Source: CAD feature listing. Evaluate the final solid. Frame: model axes, mm. A direction names the side the tool comes from. Round coordinates to 2 decimals unless told otherwise and drop trailing zeros. Loops run counter-clockwise (first coordinate to the right, second up) from the corner with the lowest first, then second, coordinate; pieces in that order, holes last. Notation, with made-up numbers: M -17.5,-14.75 L 40.5,-14.75 A20 ccw 40.5,17.25 Z; hole C 22,-22.75 d8. An arc over 180 degrees is marked long. Write each question's results on one line, items separated by ' | '. Start each with the question number.
1. Set-up query: faces 1 (the flat face through (6, -61.413, -4)), 2 (the flat face through (12, 36.087, -1)), 3 (the flat face through (-9.516, -25, 4)). Return all of +Z, -Z, +X, -X, +Y, -Y with unobstructed straight access to the full face (end or side cutting, diameter ignored); none if empty.
2. Draft query along Z for faces 4 (the flat face through (5.106, -63.857, 4.056)), 5 (the flat face through (20.484, -55, 7)), 6 (the flat face through (5.694, -19.969, 3.944)). Return one class per face: released by +Z, released by -Z, zero draft, split by the parting line, or undercut.
3. Ray query, line 1 (Y direction, x = -7, z = -0.25); line 2 (Y direction, x = 11.5, z = -1.5); line 3 (X direction, y = -0.5, z = -0.5). Return the intervals inside material, ascending.
4. Section C-C on y = 10.5. Output: boundary loops of the cut face in (x, z), and give its area (3 significant figures).
5. Section D-D on x = -4. Give the number of separate pieces and of enclosed holes in the cut face, and give its area (3 significant figures).
6. Section B-B on x = -10.5. Output: boundary loops of the cut face in (y, z), and give its area (3 significant figures).
7. Contact query for flat-ended pins moving along their axis: pin 1 Ø6.5 at (y, z) = (7.5, 4) entering from -X; pin 2 Ø12.5 at (x, y) = (12.5, -22) entering from -Z; pin 3 Ø6.5 at (y, z) = (-25.5, 5.5) entering from +X. Output: stop coordinate, or through.
8. Section A-A on z = -3.25. Output: boundary loops of the cut face in (x, y).
from build123d import *

# Parameters (mm, degrees)
SKETCH1_W               = 54
SKETCH1_H               = 104
SKETCH1_W_2             = 30
SKETCH1_H_2             = 80
BOSS_EXTRUDE1_DEPTH     = 8
CHAMFER1_SIZE           = 8
SKETCH2_W               = 54
SKETCH2_H               = 104
SKETCH2_W_2             = 50
SKETCH2_H_2             = 100
BOSS_EXTRUDE2_DEPTH     = 2
SKETCH3_W               = 44
SKETCH3_H               = 94
SKETCH3_W_2             = 41
SKETCH3_H_2             = 91
BOSS_EXTRUDE3_DEPTH     = 9
CUT_EXTRUDE1_REACH      = 106.581
SKETCH4_W               = 17
SKETCH4_H               = 1
CUT_EXTRUDE2_DEPTH      = 110.326033519
CUT_EXTRUDE2_DEPTH_BACK = 2
BOSS_EXTRUDE4_REACH     = 82.357


with BuildPart() as part:
    # Sketch1 → Boss-Extrude1 (new body)
    with BuildSketch(Plane.XY):
        with Locations((5.483558994, -15.912959381)):
            Rectangle(SKETCH1_W, SKETCH1_H)
        with Locations((5.483558994, -15.912959381)):
            Rectangle(SKETCH1_W_2, SKETCH1_H_2, mode=Mode.SUBTRACT)
    extrude(amount=BOSS_EXTRUDE1_DEPTH)

    # Chamfer1
    chamfer1_edges = [part.edges().sort_by_distance(p)[0] for p in [
        (-21.516441006, -15.912959381, 8),
        (5.483558994, 36.087040619, 8),
        (32.483558994, -15.912959381, 8),
        (5.483558994, -67.912959381, 8),
    ]]
    chamfer(chamfer1_edges, length=CHAMFER1_SIZE - 0.0001)  # a hair under: the kernel refuses the full size

    # Sketch2 → Boss-Extrude2 (add)
    with BuildSketch(Plane(origin=(0, 0, 0), x_dir=(-1, 0, 0), z_dir=(0, 0, -1))):
        with Locations((-5.483558994, -15.912959381)):
            Rectangle(SKETCH2_W, SKETCH2_H)
        with Locations((-5.483558994, -15.912959381)):
            Rectangle(SKETCH2_W_2, SKETCH2_H_2, mode=Mode.SUBTRACT)
    extrude(amount=BOSS_EXTRUDE2_DEPTH)

    # Sketch3 → Boss-Extrude3 (add)
    with BuildSketch(Plane(origin=(0, 0, 0), x_dir=(-1, 0, 0), z_dir=(0, 0, -1))):
        with Locations((-5.483558994, -15.912959381)):
            Rectangle(SKETCH3_W, SKETCH3_H)
        with Locations((-5.483558994, -15.912959381)):
            Rectangle(SKETCH3_W_2, SKETCH3_H_2, mode=Mode.SUBTRACT)
    extrude(amount=BOSS_EXTRUDE3_DEPTH)

    # Sketch4 → Cut-Extrude1 (cut, up to next)
    with BuildSketch(Plane(origin=(0, 31.087040619, 0), x_dir=(1, 0, 0), z_dir=(0, 1, 0)), mode=Mode.PRIVATE) as cut_extrude1_sk1:
        with Locations((5.483558994, 8.5)):
            Rectangle(SKETCH4_W, SKETCH4_H)
    cut_extrude1_tool1 = extrude(cut_extrude1_sk1.sketch, amount=-CUT_EXTRUDE1_REACH, mode=Mode.PRIVATE) & part.part
    add(cut_extrude1_tool1.solids().sort_by_distance((5.483559, 31.087041, -8.5))[0], mode=Mode.SUBTRACT)

    # Sketch5 → Cut-Extrude2 (cut, two sides: drawn at the far end of the back side and taken through both)
    with BuildSketch(Plane(origin=(0, 36.087040619, 0), x_dir=(1, 0, 0), z_dir=(0, 1, 0)).offset(-CUT_EXTRUDE2_DEPTH_BACK)):
        with BuildLine():
            Line((-76.690196685, 38.800488397), (-2.516441006, 2))
            ThreePointArc((-2.516441006, 2), (5.483558994, 0.124515497), (13.483558994, 2))
            Line((13.483558994, 2), (87.657314674, 38.800488397))
            Line((87.657314674, 38.800488397), (87.657314674, 204.402686182))
            Line((87.657314674, 204.402686182), (-76.690196685, 204.402686182))
            Line((-76.690196685, 204.402686182), (-76.690196685, 38.800488397))
        make_face()
    extrude(amount=CUT_EXTRUDE2_DEPTH + CUT_EXTRUDE2_DEPTH_BACK, mode=Mode.SUBTRACT)

    # Sketch6 → Boss-Extrude4 (add, up to next)
    with BuildSketch(Plane.ZY.offset(-20.483558994), mode=Mode.PRIVATE) as boss_extrude4_sk1:
        Polygon((0, -55.912959381), (8, -47.912959381), (8, -50.741386506), (2.828427125, -55.912959381), align=None)
    boss_extrude4_tool1 = extrude(boss_extrude4_sk1.sketch, amount=BOSS_EXTRUDE4_REACH, mode=Mode.PRIVATE) - part.part
    # Sketch6 → Boss-Extrude4 (add, up to next)
    with BuildSketch(Plane.ZY.offset(-20.483558994), mode=Mode.PRIVATE) as boss_extrude4_sk2:
        Polygon((0, -50.741386506), (8, -42.741386506), (8, -39.912959381), (0, -47.912959381), align=None)
    boss_extrude4_tool2 = extrude(boss_extrude4_sk2.sketch, amount=BOSS_EXTRUDE4_REACH, mode=Mode.PRIVATE) - part.part
    # Sketch6 → Boss-Extrude4 (add, up to next)
    with BuildSketch(Plane.ZY.offset(-20.483558994), mode=Mode.PRIVATE) as boss_extrude4_sk3:
        Polygon((0, -42.741386506), (0, -39.912959381), (8, -31.912959381), (8, -34.741386506), align=None)
    boss_extrude4_tool3 = extrude(boss_extrude4_sk3.sketch, amount=BOSS_EXTRUDE4_REACH, mode=Mode.PRIVATE) - part.part
    # Sketch6 → Boss-Extrude4 (add, up to next)
    with BuildSketch(Plane.ZY.offset(-20.483558994), mode=Mode.PRIVATE) as boss_extrude4_sk4:
        Polygon((0, -34.741386506), (0, -31.912959381), (8, -23.912959381), (8, -26.741386506), align=None)
    boss_extrude4_tool4 = extrude(boss_extrude4_sk4.sketch, amount=BOSS_EXTRUDE4_REACH, mode=Mode.PRIVATE) - part.part
    # Sketch6 → Boss-Extrude4 (add, up to next)
    with BuildSketch(Plane.ZY.offset(-20.483558994), mode=Mode.PRIVATE) as boss_extrude4_sk5:
        Polygon((0, -26.741386506), (0, -23.912959381), (8, -15.912959381), (8, -18.741386506), align=None)
    boss_extrude4_tool5 = extrude(boss_extrude4_sk5.sketch, amount=BOSS_EXTRUDE4_REACH, mode=Mode.PRIVATE) - part.part
    # Sketch6 → Boss-Extrude4 (add, up to next)
    with BuildSketch(Plane.ZY.offset(-20.483558994), mode=Mode.PRIVATE) as boss_extrude4_sk6:
        Polygon((0, -18.741386506), (0, -15.912959381), (8, -7.912959381), (8, -10.741386506), align=None)
    boss_extrude4_tool6 = extrude(boss_extrude4_sk6.sketch, amount=BOSS_EXTRUDE4_REACH, mode=Mode.PRIVATE) - part.part
    # Sketch6 → Boss-Extrude4 (add, up to next)
    with BuildSketch(Plane.ZY.offset(-20.483558994), mode=Mode.PRIVATE) as boss_extrude4_sk7:
        Polygon((0, -10.741386506), (0, -7.912959381), (8, 0.087040619), (8, -2.741386506), align=None)
    boss_extrude4_tool7 = extrude(boss_extrude4_sk7.sketch, amount=BOSS_EXTRUDE4_REACH, mode=Mode.PRIVATE) - part.part
    # Sketch6 → Boss-Extrude4 (add, up to next)
    with BuildSketch(Plane.ZY.offset(-20.483558994), mode=Mode.PRIVATE) as boss_extrude4_sk8:
        Polygon((0, -2.741386506), (0, 0.087040619), (8, 8.087040619), (8, 5.258613494), align=None)
    boss_extrude4_tool8 = extrude(boss_extrude4_sk8.sketch, amount=BOSS_EXTRUDE4_REACH, mode=Mode.PRIVATE) - part.part
    # Sketch6 → Boss-Extrude4 (add, up to next)
    with BuildSketch(Plane.ZY.offset(-20.483558994), mode=Mode.PRIVATE) as boss_extrude4_sk9:
        Polygon((0, 5.258613494), (0, 8.087040619), (8, 16.087040619), (8, 13.258613494), align=None)
    boss_extrude4_tool9 = extrude(boss_extrude4_sk9.sketch, amount=BOSS_EXTRUDE4_REACH, mode=Mode.PRIVATE) - part.part
    # Sketch6 → Boss-Extrude4 (add, up to next)
    with BuildSketch(Plane.ZY.offset(-20.483558994), mode=Mode.PRIVATE) as boss_extrude4_sk10:
        Polygon((8, 24.087040619), (8, 21.258613494), (0, 13.258613494), (0, 20.302668178), (3.784372441, 24.087040619), align=None)
    boss_extrude4_tool10 = extrude(boss_extrude4_sk10.sketch, amount=BOSS_EXTRUDE4_REACH, mode=Mode.PRIVATE) - part.part
    add(boss_extrude4_tool1.solids().sort_by_distance((20.483559, -52.569452, 4.656493))[0])
    add(boss_extrude4_tool2.solids().sort_by_distance((20.483559, -45.327173, 4))[0])
    add(boss_extrude4_tool3.solids().sort_by_distance((20.483559, -37.327173, 4))[0])
    add(boss_extrude4_tool4.solids().sort_by_distance((20.483559, -29.327173, 4))[0])
    add(boss_extrude4_tool5.solids().sort_by_distance((20.483559, -21.327173, 4))[0])
    add(boss_extrude4_tool6.solids().sort_by_distance((20.483559, -13.327173, 4))[0])
    add(boss_extrude4_tool7.solids().sort_by_distance((20.483559, -5.327173, 4))[0])
    add(boss_extrude4_tool8.solids().sort_by_distance((20.483559, 2.672827, 4))[0])
    add(boss_extrude4_tool9.solids().sort_by_distance((20.483559, 10.672827, 4))[0])
    add(boss_extrude4_tool10.solids().sort_by_distance((20.483559, 19.898628, 3.514255))[0])


solid = part.part
Taken from the geometry:
1) face 1: -Z | face 2: +Z, -Z, +X, -X, +Y | face 3: none
2) face 4: released by +Z | face 5: zero draft | face 6: undercut
3) line 1: -67.91 to -65.91, -62.91 to -61.41, 29.59 to 31.09, 34.09 to 36.09 | line 2: -67.91 to -65.91, -62.91 to -61.41, 29.59 to 31.09 | line 3: -21.52 to -19.52, -16.52 to -15.02, 25.98 to 27.48, 30.48 to 32.48
4) outline: M -21.52,-2 L -19.52,-2 L -19.52,0 L -16.52,0 L -16.52,-9 L -15.02,-9 L -15.02,0 L -9.52,0 L -9.52,2.41 L 20.48,2.41 L 20.48,0 L 25.98,0 L 25.98,-9 L 27.48,-9 L 27.48,0 L 30.48,0 L 30.48,-2 L 32.48,-2 L 32.48,0 L 24.48,8 L 20.48,8 L 20.48,5.24 L -9.52,5.24 L -9.52,8 L -13.52,8 L -21.52,0 Z | area: 248 mm^2
5) separate pieces: 10 | enclosed holes: 0 | area: 410 mm^2
6) outline: M -67.91,-2 L -65.91,-2 L -65.91,0 L -62.91,0 L -62.91,-9 L -61.41,-9 L -61.41,0 L 29.59,0 L 29.59,-9 L 31.09,-9 L 31.09,0 L 34.09,0 L 34.09,-2 L 36.09,-2 L 36.09,0 L 28.09,8 L -59.91,8 L -67.91,0 Z | area: 803 mm^2
7) pin 1: x = -20.77 | pin 2: z = 0 | pin 3: x = 30.23
8) outline: M -16.52,-62.91 L 27.48,-62.91 L 27.48,31.09 L -16.52,31.09 Z; hole M -15.02,-61.41 L 25.98,-61.41 L 25.98,29.59 L -15.02,29.59 Z
